For this review, take the finished solid that the model builds, in its own axes (mm). Face numbers are marked on the shaded views. A direction names the side the tool comes from. Coordinates: 2 decimals unless noted, no trailing zeros. Loops run counter-clockwise (first coordinate to the right, second up) from the corner with the lowest first, then second, coordinate; pieces in that order, holes last. Notation, with made-up numbers: (50, 12) - (76, 12) arc R11 cw to (76, 16) - close; hole circle Ø10 at (74.25, 66.5). An arc over 180 degrees is marked (long way). One line per item, written item: value. Start each with the question number.
1. Take a section at C-C, the plane z = 1.55. State the section outline as (x, y) points.
2. Insertion check: pin 1 (1 mm diameter, centred on y = 7.5, z = 1.5, fed in from -X); pin 2 (1.5 mm diameter, centred on x = 4, z = 3, fed in from -Y); pin 3 (0.7 mm diameter, centred on y = 8, z = 2.5, fed in from +X); pin 4 (0.6 mm diameter, centred on x = 17, z = 2, fed in from +Y). Each pin has a flat end and moves straight along its axis. Give the tip position at first contact, or say it passes through.
3. Take a section at D-D, the plane y = 9.5. State the section outline as (x, z) points, and give its area (3 significant figures).
4. For the marked faces 1, 2, 3, 4 and 5, list the 3-axis set-ups (+Z, -Z, +X, -X, +Y, -Y) from which the entire face can be reached by the end or side of a thin tool; tool diameter is ignored.
5. The part is to be moulded in two halves that separate along X. For the marked faces 6, 7 and 8, say which applies: released by +X, released by -X, zero draft, split by the parting line, or undercut.
6. To check wall thickness, follow line 1 (Y direction, x = 16.5, z = 0.65) (3 decimals); line 2 (X direction, y = 5.75, z = 2.5); line 3 (Y direction, x = 11, z = 2.6). State the ranges of each line that lie inside material, in increasing order. Write a range as from..to.
7. Take a section at B-B, the plane y = 1.5. State the section outline as (x, z) points (3 decimals).
8. Take a section at A-A, the plane x = 16.5. State the section outline as (y, z) points (3 decimals), and give its area (3 significant figures).
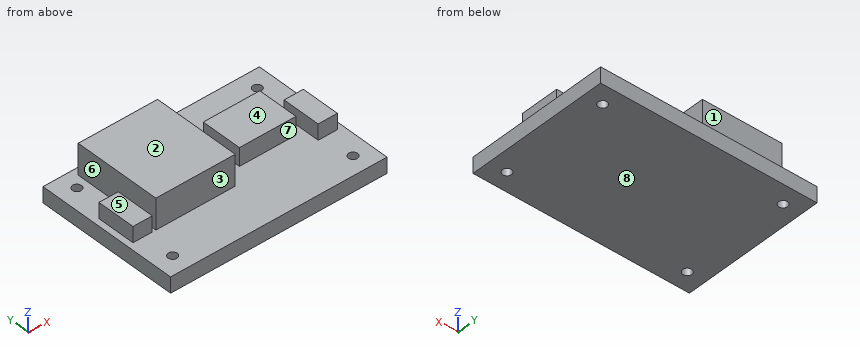
```python
from build123d import *

# Parameters (mm, degrees)
SKIZZE1_W                       = 18
SKIZZE1_H                       = 12
PLATINE_DEPTH                   = 1.3
SKIZZE2_W                       = 6.6
SKIZZE2_H                       = 7.3
AUFSATZ_LINEAR_AUSTRAGEN2_DEPTH = 2.55
SKIZZE3_W                       = 4.7
SKIZZE3_H                       = 3.4
AUFSATZ_LINEAR_AUSTRAGEN3_DEPTH = 1.5
SKIZZE4_R                       = 0.375
SCHNITT_LINEAR_AUSTRAGEN1_DEPTH = 22.783078295
SKIZZE5_W                       = 1.6
SKIZZE5_H                       = 3.2
AUFSATZ_LINEAR_AUSTRAGEN4_DEPTH = 1.3


with BuildPart() as part:
    # Skizze1 → Platine (new body)
    with BuildSketch(Plane.XY):
        with Locations((9, 6)):
            Rectangle(SKIZZE1_W, SKIZZE1_H)
    extrude(amount=PLATINE_DEPTH)

    # Skizze2 → Aufsatz-Linear austragen2 (add)
    with BuildSketch(Plane.XY.offset(1.3)):
        with Locations((5.7, 7.75)):
            Rectangle(SKIZZE2_W, SKIZZE2_H)
    extrude(amount=AUFSATZ_LINEAR_AUSTRAGEN2_DEPTH)

    # Skizze3 → Aufsatz-Linear austragen3 (add)
    with BuildSketch(Plane.XY.offset(1.3)):
        with Locations((12.85, 7.1)):
            Rectangle(SKIZZE3_W, SKIZZE3_H)
    extrude(amount=AUFSATZ_LINEAR_AUSTRAGEN3_DEPTH)

    # Skizze4 → Schnitt-Linear austragen1 (cut, through all)
    with BuildSketch(Plane.XY.offset(1.3)):
        with Locations((1.5, 10.5)):
            Circle(SKIZZE4_R)
        with Locations(Location((16.5, 10.5, 0), (0, 0, 180))):
            Circle(SKIZZE4_R)
        with Locations((16.5, 1.5)):
            Circle(SKIZZE4_R)
        with Locations(Location((1.5, 1.5, 0), (0, 0, 180))):
            Circle(SKIZZE4_R)
    extrude(amount=-SCHNITT_LINEAR_AUSTRAGEN1_DEPTH, mode=Mode.SUBTRACT)

    # Skizze5 → Aufsatz-Linear austragen4 (add)
    with BuildSketch(Plane.XY.offset(1.3)):
        with Locations((1.3, 5.7)):
            Rectangle(SKIZZE5_W, SKIZZE5_H)
        with Locations((16.7, 5.7)):
            Rectangle(SKIZZE5_W, SKIZZE5_H)
    extrude(amount=AUFSATZ_LINEAR_AUSTRAGEN4_DEPTH)


solid = part.part
```
Solutions:
1. outline: (0.5, 4.1) - (2.1, 4.1) - (2.1, 7.3) - (0.5, 7.3) - close; (2.4, 4.1) - (9, 4.1) - (9, 11.4) - (2.4, 11.4) - close; (10.5, 5.4) - (15.2, 5.4) - (15.2, 8.8) - (10.5, 8.8) - close; (15.9, 4.1) - (17.5, 4.1) - (17.5, 7.3) - (15.9, 7.3) - close
2. pin 1: x = 0
2. pin 2: y = 4.1
2. pin 3: x = 15.2
2. pin 4: y = 7.3
3. outline: (0, 0) - (18, 0) - (18, 1.3) - (9, 1.3) - (9, 3.85) - (2.4, 3.85) - (2.4, 1.3) - (0, 1.3) - close
3. area: 40.2 mm2
4. face 1: +Z, +X, -X, +Y
4. face 2: +Z, +X, -X, +Y, -Y
4. face 3: +Z, +X, -X, -Y
4. face 4: +Z, +X, +Y, -Y
4. face 5: +Z, -X, +Y, -Y
5. face 6: undercut
5. face 7: undercut
5. face 8: zero draft
6. line 1: 0..1.125, 1.875..10.125, 10.875..12
6. line 2: 0.5..2.1, 2.4..9, 10.5..15.2, 15.9..17.5
6. line 3: 5.4..8.8
7. outline: (0, 0) - (1.125, 0) - (1.125, 1.3) - (0, 1.3) - close; (1.875, 0) - (16.125, 0) - (16.125, 1.3) - (1.875, 1.3) - close; (16.875, 0) - (18, 0) - (18, 1.3) - (16.875, 1.3) - close
8. outline: (0, 0) - (1.125, 0) - (1.125, 1.3) - (0, 1.3) - close; (1.875, 0) - (10.125, 0) - (10.125, 1.3) - (7.3, 1.3) - (7.3, 2.6) - (4.1, 2.6) - (4.1, 1.3) - (1.875, 1.3) - close; (10.875, 0) - (12, 0) - (12, 1.3) - (10.875, 1.3) - close
8. area: 17.8 mm2
